Part model, mm, in its own coordinate system. Face numbers are marked on the shaded views. Round coordinates to 2 decimals unless told otherwise and drop trailing zeros. Write each loop counter-clockwise with the first axis right and the second up, starting at its lowest first coordinate (ties: lowest second). Pieces come first, ordered by that corner, then holes. Notation, with made-up numbers: M 58,74 L 112,74 A21 ccw 112,109 Z; hole C 66.25,89.25 d10. An arc over 180 degrees is marked long. Answer as a JSON object with one key per item and string values. Group by question number.
1. Two-plate mould, pull along X, no slides. Class the marked faces 1, 2 and 3: +X half, -X half, draft (parallel to the pull), parting line (faces both ways), or undercut.
2. Band-saw the part on C-C, the plane y = -4. Write the cut outline in (x, z), plus the area to 3 significant figures.
3. Band-saw the part on B-B, the plane z = 3.2. Write the cut outline in (x, y).
4. Band-saw the part on D-D, the plane x = -12. Write the cut outline in (y, z).
5. Band-saw the part on A-A, the plane y = 3. Write the cut outline in (x, z).
6. Drop flat-ended pins along their axis: pin 1 (1 mm diameter, centred on x = 12.5, y = -9, fed in from -Z); pin 2 (10.5 mm diameter, centred on x = 13.49, y = 0.87, fed in from +Z); pin 3 (1 mm diameter, centred on x = -39.5, z = 2, fed in from +Y); pin 4 (1.5 mm diameter, centred on x = -38, z = 2, fed in from +Y). Give the stop position or say it passes through.
7. Drill centre lines: line 1 (X direction, y = 1.5, z = 3.3); line 2 (Z direction, x = 11, y = 9.5); line 3 (X direction, y = 8, z = 3.1). Where is each one in solid material? Low to high. Write a range as from..to.
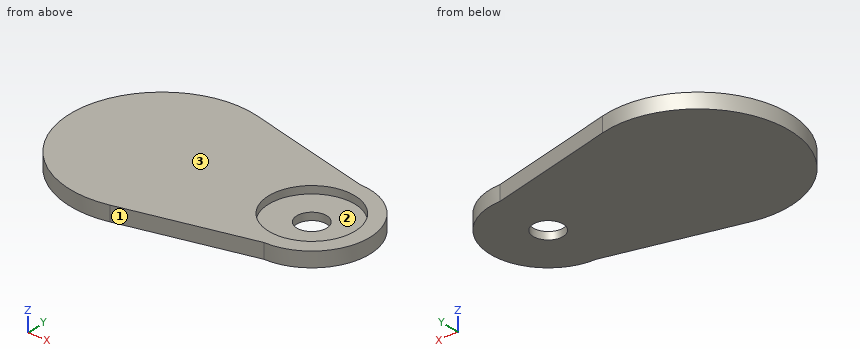
from build123d import *

# Parameters (mm, degrees)
EXTRUDE_1_DEPTH     = 4
SKETCH_2_R          = 11.5
CUT_EXTRUDE_1_DEPTH = 2
SKETCH_3_R          = 4
CUT_EXTRUDE_2_DEPTH = 2


with BuildPart() as part:
    # 草图1 → 凸台-拉伸1 (new body)
    with BuildSketch(Plane.XY):
        with BuildLine():
            Line((13.490639399, 16.366658186), (-20.728829372, 24.674964692))
            ThreePointArc((-20.728829372, 24.674964692), (-51.009360601, 0.866658186), (-20.728829372, -22.941648321))
            Line((-20.728829372, -22.941648321), (13.490639399, -14.633341814))
            ThreePointArc((13.490639399, -14.633341814), (28.990639399, 0.866658186), (13.490639399, 16.366658186))
        make_face()
    extrude(amount=EXTRUDE_1_DEPTH)

    # 草图2 → 切除-拉伸1 (cut)
    with BuildSketch(Plane.XY.offset(4)):
        with Locations((13.490639399, 0.866658186)):
            Circle(SKETCH_2_R)
    extrude(amount=-CUT_EXTRUDE_1_DEPTH, mode=Mode.SUBTRACT)

    # 草图3 → 切除-拉伸2 (cut)
    with BuildSketch(Plane.XY.offset(2)):
        with Locations((13.490639399, 0.866658186)):
            Circle(SKETCH_3_R)
    extrude(amount=-CUT_EXTRUDE_2_DEPTH, mode=Mode.SUBTRACT)


solid = part.part
Worked answers:
{
 "1": {"face 1": "+X half", "face 2": "undercut", "face 3": "draft"},
 "2": {"outline": "M -50.52,0 L 28.21,0 L 28.21,4 L 23.91,4 L 23.91,2 L 3.07,2 L 3.07,4 L -50.52,4 Z", "area": "273 mm^2"},
 "3": {"outline": "M -20.73,-22.94 L 13.49,-14.63 A15.5 ccw 13.49,16.37 L -20.73,24.67 A24.5 ccw long Z; hole C 13.49,0.87 d23"},
 "4": {"outline": "M -20.82,0 L 22.56,0 L 22.56,4 L -20.82,4 Z"},
 "5": {"outline": "M -50.92,0 L 10.11,0 L 10.11,2 L 2.19,2 L 2.19,4 L -50.92,4 Z; M 16.87,0 L 28.84,0 L 28.84,4 L 24.79,4 L 24.79,2 L 16.87,2 Z"},
 "6": {"pin 1": "stops at z = 0", "pin 2": "stops at z = 2", "pin 3": "stops at y = 21.94", "pin 4": "stops at y = 22.89"},
 "7": {"line 1": "x = -51..2.01, 24.97..28.98", "line 2": "z = 0..2", "line 3": "x = -49.95..4.47, 22.51..27.25"}
}
